from build123d import *

# Parameters (mm, degrees)
F1_DEPTH = 3
F2_R     = 4
F3_DEPTH = 10
F3_TAPER = 21
F5_COUNT = 4
F5_ANGLE = 270
F7_DEPTH = 10
F8_W     = 40
F8_H     = 40
F9_DEPTH = 3
F10_SIZE = 2


with BuildPart() as f1:
    # F0 (on Front) → F1 (new body)
    with BuildSketch(Plane.XZ):
        with BuildLine():
            ThreePointArc((32, 27), (30.5355339059, 30.5355339059), (27, 32))
            Line((27, 32), (-27, 32))
            ThreePointArc((-27, 32), (-30.5355339059, 30.5355339059), (-32, 27))
            Line((-32, 27), (-32, -27))
            ThreePointArc((-32, -27), (-30.5355339059, -30.5355339059), (-27, -32))
            Line((-27, -32), (27, -32))
            ThreePointArc((27, -32), (30.5355339059, -30.5355339059), (32, -27))
            Line((32, -27), (32, 27))
        make_face()
    extrude(amount=F1_DEPTH)

    # F2 (on face) → F3 (join)
    with BuildSketch(Plane.XZ.offset(3)):
        with Locations((-24.8786796564, 24.8786796564)):
            Circle(F2_R)
    extrude(amount=F3_DEPTH, taper=F3_TAPER)

    # F5: F1 ×4 about axis
    f5_axis = Axis((0, -16.6125968099, 0), (0, -1, 0))


with BuildPart() as f1_1:
    add(f1.part)
    for i in range(1, F5_COUNT):
        add(f1.part.rotate(f5_axis, i * F5_ANGLE / (F5_COUNT - 1)))

    # F6 (on face) → F7 (join)
    with BuildSketch(Plane.XZ.offset(3)):
        with BuildLine():
            ThreePointArc((-27, 36), (-33.3639610307, 33.3639610307), (-36, 27))
            Line((-36, 27), (-36, -27))
            ThreePointArc((-36, -27), (-33.3639610307, -33.3639610307), (-27, -36))
            Line((-27, -36), (27, -36))
            ThreePointArc((27, -36), (33.3639610307, -33.3639610307), (36, -27))
            Line((36, -27), (36, 27))
            ThreePointArc((36, 27), (33.3639610307, 33.3639610307), (27, 36))
            Line((27, 36), (-27, 36))
        make_face()
        with BuildLine():
            ThreePointArc((27, 32), (30.5355339059, 30.5355339059), (32, 27))
            Line((32, 27), (32, -27))
            ThreePointArc((32, -27), (30.5355339059, -30.5355339059), (27, -32))
            Line((27, -32), (-27, -32))
            ThreePointArc((-27, -32), (-30.5355339059, -30.5355339059), (-32, -27))
            Line((-32, -27), (-32, 27))
            ThreePointArc((-32, 27), (-30.5355339059, 30.5355339059), (-27, 32))
            Line((-27, 32), (27, 32))
        make_face(mode=Mode.SUBTRACT)
    extrude(amount=-F7_DEPTH)

    # F8 (on face) → F9 (cut)
    with BuildSketch(Plane.XZ.offset(3)):
        Rectangle(F8_W, F8_H)
    extrude(amount=-F9_DEPTH, mode=Mode.SUBTRACT)

    # F10
    f10_edges = [f1_1.edges().sort_by_distance(p)[0] for p in [
        (0, 7, -32),
        (0, 0, -20),
        (20, 0, 0),
        (-20, 0, 0),
        (0, 0, 20),
    ]]
    chamfer(f10_edges, length=F10_SIZE)


solid = f1_1.part
Input: part model. Units: mm. Frame: model coordinates. A direction names the side the tool comes from. Round coordinates to 2 decimals unless told otherwise and drop trailing zeros. Loops run counter-clockwise (first coordinate to the right, second up) from the corner with the lowest first, then second, coordinate; pieces in that order, holes last. Notation, with made-up numbers: (11, 49.25) -> (55, 49.25) arc R16 cw to (55, 59.25) -> close; hole circle Ø6 at (10.25, 57). An arc over 180 degrees is marked (long way). Answer as a JSON object with one key per item and string values. Group by question number.
1) Pin query (flat end, axial travel): pin 1 (19 mm diameter, centred on x = -14, z = -3, fed in from +Y). Return the tip coordinate at first contact, or that it passes through.
2) Section query D-D on y = -9.5. Output: boundary loops of the cut face in (x, z).
3) Reachability of faces 1 (the conical face through (-31.031, 5.764, -31.12)), 2 (the flat face through (-25, -3, 1)), 3 (the cylindrical face through (-33.294, 1.93, 33.434)) from +Z, -Z, +X, -X, +Y, -Y: full face, straight path, thin tool, end or side. Return the list, or none.
4) Section query A-A on z = 17.5. Output: boundary loops of the cut face in (x, y).
5) Section query B-B on y = 3. Output: boundary loops of the cut face in (x, z).
6) Ray query, L1, parallel to X at y = 0.5, z = -6.5; L2, parallel to Y at x = 30.5, z = -5. Return the intervals inside material, ascending.
7) Section query C-C on x = -12. Output: boundary loops of the cut face in (y, z).
8) Draft query along Z for faces 4 (the flat face through (0, 2, 32)), 5 (the conical face through (31.12, 5.764, -31.031)), 6 (the cylindrical face through (33.434, 1.93, 33.294)), 7 (the flat face through (36, 2, 0)). Return one class per face: +Z half, -Z half, draft (parallel to the pull), parting line (faces both ways), or undercut.
Reply:
{
 "1": {"pin 1": "stops at y = 0"},
 "2": {"outline": "circle Ø3.01 at (-24.88, -24.88); circle Ø3.01 at (-24.88, 24.88); circle Ø3.01 at (24.88, -24.88); circle Ø3.01 at (24.88, 24.88)"},
 "3": {"face 1": "+Y", "face 2": "-Y", "face 3": "+Z, -X, +Y, -Y"},
 "4": {"outline": "(-36, -3) -> (-20, -3) -> (-20, -2) -> (-22, 0) -> (-32, 0) -> (-32, 5) -> (-34, 7) -> (-36, 7) -> close; (20, -3) -> (36, -3) -> (36, 7) -> (34, 7) -> (32, 5) -> (32, 0) -> (22, 0) -> (20, -2) -> close"},
 "5": {"outline": "(-36, -27) arc R9 ccw to (-27, -36) -> (27, -36) arc R9 ccw to (36, -27) -> (36, 27) arc R9 ccw to (27, 36) -> (-27, 36) arc R9 ccw to (-36, 27) -> close; hole (-32, -27) arc R5 ccw to (-27, -32) -> (27, -32) arc R5 ccw to (32, -27) -> (32, 27) arc R5 ccw to (27, 32) -> (-27, 32) arc R5 ccw to (-32, 27) -> close"},
 "6": {"L1": "x = -36 to -32, 32 to 36", "L2": "y = -3 to 0"},
 "7": {"outline": "(-3, -36) -> (7, -36) -> (7, -34) -> (5, -32) -> (0, -32) -> (0, -22) -> (-2, -20) -> (-3, -20) -> close; (-3, 20) -> (-2, 20) -> (0, 22) -> (0, 32) -> (5, 32) -> (7, 34) -> (7, 36) -> (-3, 36) -> close"},
 "8": {"face 4": "undercut", "face 5": "undercut", "face 6": "+Z half", "face 7": "draft"}
}
